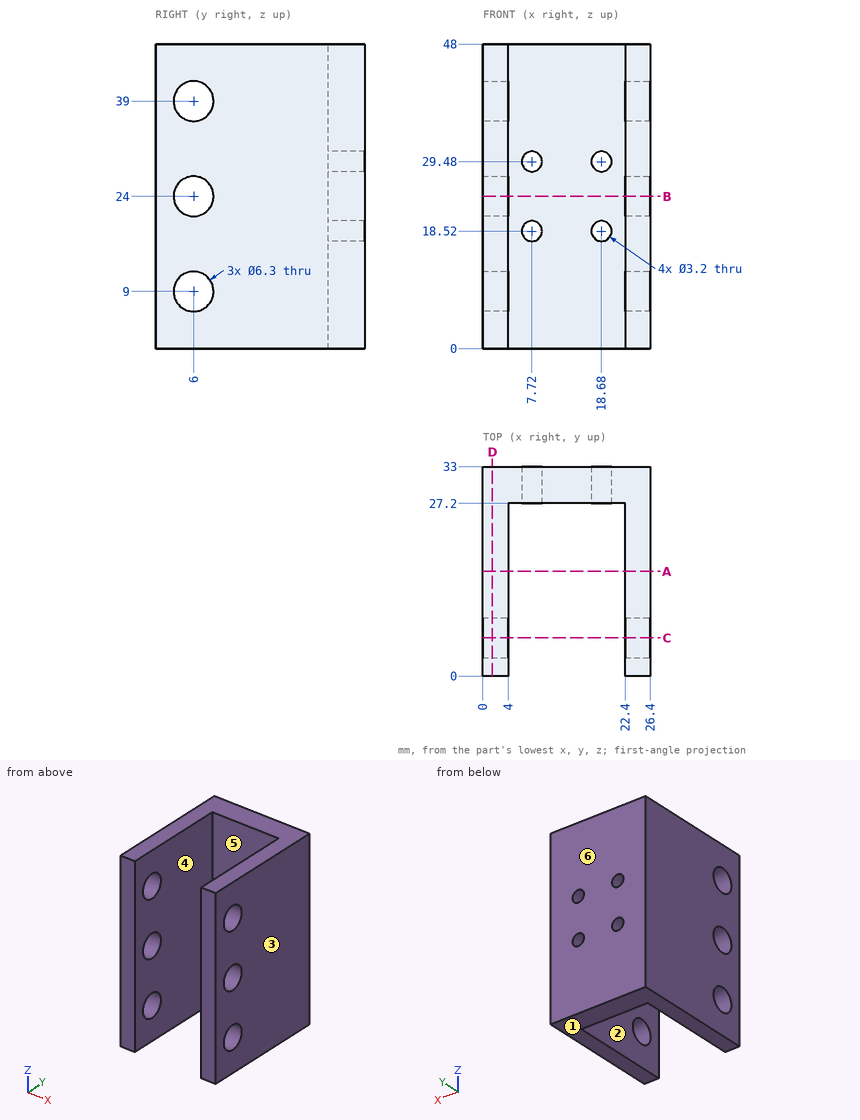
Answer from the drawing. Dimensions are ordinates in mm from the lowest x, y and z of the part. A direction names the side the tool comes from. Coordinates: 2 decimals unless noted, no trailing zeros. Loops run counter-clockwise (first coordinate to the right, second up) from the corner with the lowest first, then second, coordinate; pieces in that order, holes last.
1) Section C-C (y = 6) is taken. Give the number of separate pieces and of enclosed holes in the cut face, plus the area to 3 significant figures.
Results:
separate pieces: 8
enclosed holes: 0
area: 233 mm2
2) For the marked faces 5 and 6, determine the directions among +Z, -Z, +X, -X, +Y, -Y from which every point of the face is accessible in a straight line to the end or side of a thin tool.
Results:
face 5: +Z, -Z, -Y
face 6: +Z, -Z, +X, -X, +Y
3) Flat-ended cylindrical pins translate along their axes: pin 1 (10 mm diameter, centred on y = 6, z = 39, fed in from -X); pin 2 (5.5 mm diameter, centred on x = 9.5, z = 31.5, fed in from -Y). Find the tip coordinate at first contact, or state that the pin passes through.
Results:
pin 1: stops at x = 0
pin 2: stops at y = 27.2
4) For a pull along X with two mould halves and no side action, classify the marked faces 1, 2, 3 and 4 as +X half, -X half, draft (parallel to the pull), parting line (faces both ways), or undercut.
Results:
face 1: draft
face 2: undercut
face 3: +X half
face 4: undercut
5) Section A-A (y = 16.5) is taken. Give the vertices of the cut face in (x, z), plus the area to 3 significant figures.
Results:
outline: (0, 0) - (4, 0) - (4, 48) - (0, 48) - close; (22.4, 0) - (26.4, 0) - (26.4, 48) - (22.4, 48) - close
area: 384 mm2
6) Section D-D (x = 1.5) is taken. Give the vertices of the cut face in (y, z), plus the area to 3 significant figures.
Results:
outline: (0, 0) - (33, 0) - (33, 48) - (0, 48) - close; hole circle Ø6.3 at (6, 9); hole circle Ø6.3 at (6, 24); hole circle Ø6.3 at (6, 39)
area: 1,490 mm2
7) Consider probe 1 along Y at (x, z) = (1.55, 24); probe 2 along X at (y, z) = (17.5, 26.5); probe 3 along X at (y, z) = (27.5, 19). Determine where each line is inside the solid, lowest interval first.
Results:
probe 1: y = 0 to 2.85, 9.15 to 33
probe 2: x = 0 to 4, 22.4 to 26.4
probe 3: x = 0 to 6.19, 9.25 to 17.15, 20.21 to 26.4
8) Section B-B (z = 24) is taken. Give the vertices of the cut face in (x, y), plus the area to 3 significant figures.
Results:
outline: (0, 0) - (4, 0) - (4, 2.85) - (0, 2.85) - close; (0, 9.15) - (4, 9.15) - (4, 27.2) - (22.4, 27.2) - (22.4, 9.15) - (26.4, 9.15) - (26.4, 33) - (0, 33) - close; (22.4, 0) - (26.4, 0) - (26.4, 2.85) - (22.4, 2.85) - close
area: 320 mm2
